The listing builds one solid part. Answer for the finished solid, in the listing's coordinates (mm). Face numbers are marked on the shaded views. A direction names the side the tool comes from. Round coordinates to 2 decimals unless told otherwise and drop trailing zeros. Write each loop counter-clockwise with the first axis right and the second up, starting at its lowest first coordinate (ties: lowest second). Pieces come first, ordered by that corner, then holes. Notation, with made-up numbers: (21.5, 22.25) - (54.5, 22.25) arc R23 cw to (54.5, 43.25) - close; hole circle Ø6 at (82.25, 17.25). An arc over 180 degrees is marked (long way). Return JSON: item names as keys, results as strings. Group by question number.
from build123d import *

# Parameters (mm, degrees)
SKETCH1_W                       = 27.7
SKETCH1_H                       = 41.5
BOSS_EXTRUDE1_DEPTH             = 10
CUT_EXTRUDE2_DEPTH              = 27.877220838
CUT_EXTRUDE2_DEPTH_BACK         = 27.877220838
SKETCH2_R                       = 1.65
BOSS_EXTRUDE2_REACH             = 28.877
SKETCH3_R                       = 1.25
BOSS_EXTRUDE2_DIRECTION_2_REACH = 28.877
CUT_EXTRUDE3_START              = -7
SKETCH4_R                       = 1.25
CUT_EXTRUDE3_DEPTH              = 7
SKETCH6_R                       = 1.25
CUT_EXTRUDE5_DEPTH              = 10
SKETCH5_R                       = 1.25
CUT_EXTRUDE4_DEPTH              = 51.438166105
FILLET1_R                       = 2


with BuildPart() as part:
    # Sketch1 → Boss-Extrude1 (new body)
    with BuildSketch(Plane.XY):
        Rectangle(SKETCH1_W, SKETCH1_H)
    extrude(amount=BOSS_EXTRUDE1_DEPTH)

    # Sketch2 → Cut-Extrude2 (cut, two sides: drawn at the far end of the back side and taken through both)
    with BuildSketch(Plane(origin=(0, 0, 0), x_dir=(0, 0, -1), z_dir=(1, 0, 0)).offset(-CUT_EXTRUDE2_DEPTH_BACK)):
        with Locations((-4, 12.5)):
            Circle(SKETCH2_R)
        with Locations((-4, -12.5)):
            Circle(SKETCH2_R)
    extrude(amount=CUT_EXTRUDE2_DEPTH + CUT_EXTRUDE2_DEPTH_BACK, mode=Mode.SUBTRACT)

    # Boss-Extrude2: up to this face of the body (flat: up to its plane)
    boss_extrude2_end = Plane(part.part.faces().sort_by_distance((-13.85, 0, 5.042991276))[0])
    # Sketch3 → Boss-Extrude2 (add, up to the picked face)
    with BuildSketch(Plane(origin=(0, 0, 0), x_dir=(0, 0, -1), z_dir=(1, 0, 0)), mode=Mode.PRIVATE) as boss_extrude2_sk1:
        Polygon((-15.5, -14.05), (-10, -14.05), (-10, 3.45), (-20.188333796, 3.45), align=None)
    boss_extrude2_tool1 = split(extrude(boss_extrude2_sk1.sketch, amount=-BOSS_EXTRUDE2_REACH, mode=Mode.PRIVATE), bisect_by=boss_extrude2_end, keep=Keep.BOTH, mode=Mode.PRIVATE)
    # Sketch3 → Boss-Extrude2 (add, up to the picked face)
    with BuildSketch(Plane(origin=(0, 0, 0), x_dir=(0, 0, -1), z_dir=(1, 0, 0)), mode=Mode.PRIVATE) as boss_extrude2_sk2:
        with BuildLine():
            Line((-20.188333796, 3.45), (-10, 3.45))
            Line((-10, 3.45), (-10, 20.75))
            Line((-10, 20.75), (-34.754426044, 8.380905804))
            ThreePointArc((-34.754426044, 8.380905804), (-35.758048448, 2.871948872), (-30.188333796, 3.45))
            Line((-30.188333796, 3.45), (-20.188333796, 3.45))
        make_face()
        with Locations(Location((-33.19, 5.25, 0), (0, 0, 90))):
            Circle(SKETCH3_R, mode=Mode.SUBTRACT)
    boss_extrude2_tool2 = split(extrude(boss_extrude2_sk2.sketch, amount=-BOSS_EXTRUDE2_REACH, mode=Mode.PRIVATE), bisect_by=boss_extrude2_end, keep=Keep.BOTH, mode=Mode.PRIVATE)
    # Sketch3 → Boss-Extrude2 (add, up to the picked face)
    with BuildSketch(Plane(origin=(0, 0, 0), x_dir=(0, 0, -1), z_dir=(1, 0, 0)), mode=Mode.PRIVATE) as boss_extrude2_sk3:
        Polygon((-10, -14.05), (-10, -20.75), (-15.5, -14.05), align=None)
    boss_extrude2_tool3 = split(extrude(boss_extrude2_sk3.sketch, amount=-BOSS_EXTRUDE2_REACH, mode=Mode.PRIVATE), bisect_by=boss_extrude2_end, keep=Keep.BOTH, mode=Mode.PRIVATE)
    add(boss_extrude2_tool1.solids().sort_by(Axis((0, -4.428377, 14.038839), (-1, 0, 0)))[0])
    add(boss_extrude2_tool2.solids().sort_by(Axis((0, 9.377547, 20.597774), (-1, 0, 0)))[0])
    add(boss_extrude2_tool3.solids().sort_by(Axis((0, -16.283333, 11.833333), (-1, 0, 0)))[0])

    # Boss-Extrude2 direction 2: up to this face of the body (flat: up to its plane)
    boss_extrude2_direction_2_end = Plane(part.part.faces().sort_by_distance((13.85, 0, 5.042991276))[0])
    # Sketch3 → Boss-Extrude2 direction 2 (add, up to the picked face)
    with BuildSketch(Plane(origin=(0, 0, 0), x_dir=(0, 0, -1), z_dir=(1, 0, 0)), mode=Mode.PRIVATE) as boss_extrude2_direction_2_sk1:
        Polygon((-15.5, -14.05), (-10, -14.05), (-10, 3.45), (-20.188333796, 3.45), align=None)
    boss_extrude2_direction_2_tool1 = split(extrude(boss_extrude2_direction_2_sk1.sketch, amount=BOSS_EXTRUDE2_DIRECTION_2_REACH, mode=Mode.PRIVATE), bisect_by=boss_extrude2_direction_2_end, keep=Keep.BOTH, mode=Mode.PRIVATE)
    # Sketch3 → Boss-Extrude2 direction 2 (add, up to the picked face)
    with BuildSketch(Plane(origin=(0, 0, 0), x_dir=(0, 0, -1), z_dir=(1, 0, 0)), mode=Mode.PRIVATE) as boss_extrude2_direction_2_sk2:
        with BuildLine():
            Line((-20.188333796, 3.45), (-10, 3.45))
            Line((-10, 3.45), (-10, 20.75))
            Line((-10, 20.75), (-34.754426044, 8.380905804))
            ThreePointArc((-34.754426044, 8.380905804), (-35.758048448, 2.871948872), (-30.188333796, 3.45))
            Line((-30.188333796, 3.45), (-20.188333796, 3.45))
        make_face()
        with Locations(Location((-33.19, 5.25, 0), (0, 0, 90))):
            Circle(SKETCH3_R, mode=Mode.SUBTRACT)
    boss_extrude2_direction_2_tool2 = split(extrude(boss_extrude2_direction_2_sk2.sketch, amount=BOSS_EXTRUDE2_DIRECTION_2_REACH, mode=Mode.PRIVATE), bisect_by=boss_extrude2_direction_2_end, keep=Keep.BOTH, mode=Mode.PRIVATE)
    # Sketch3 → Boss-Extrude2 direction 2 (add, up to the picked face)
    with BuildSketch(Plane(origin=(0, 0, 0), x_dir=(0, 0, -1), z_dir=(1, 0, 0)), mode=Mode.PRIVATE) as boss_extrude2_direction_2_sk3:
        Polygon((-10, -14.05), (-10, -20.75), (-15.5, -14.05), align=None)
    boss_extrude2_direction_2_tool3 = split(extrude(boss_extrude2_direction_2_sk3.sketch, amount=BOSS_EXTRUDE2_DIRECTION_2_REACH, mode=Mode.PRIVATE), bisect_by=boss_extrude2_direction_2_end, keep=Keep.BOTH, mode=Mode.PRIVATE)
    add(boss_extrude2_direction_2_tool1.solids().sort_by(Axis((0, -4.428377, 14.038839), (1, 0, 0)))[0])
    add(boss_extrude2_direction_2_tool2.solids().sort_by(Axis((0, 9.377547, 20.597774), (1, 0, 0)))[0])
    add(boss_extrude2_direction_2_tool3.solids().sort_by(Axis((0, -16.283333, 11.833333), (1, 0, 0)))[0])

    # Sketch4 → Cut-Extrude3 (cut)
    # profile 1 of 5: a face of its own
    with BuildSketch(Plane.ZY.offset(13.85).offset(CUT_EXTRUDE3_START)):
        with BuildLine():
            ThreePointArc((34.754426044, 8.380905804), (30.621951552, 7.628051128), (30.188333796, 3.45))
            ThreePointArc((30.188333796, 3.45), (34.123854455, 1.876883361), (36.69, 5.25))
            ThreePointArc((36.69, 5.25), (36.167036375, 7.090449517), (34.754426044, 8.380905804))
        make_face()
        with Locations(Location((33.19, 5.25, 0), (0, 0, 270))):
            Circle(SKETCH4_R, mode=Mode.SUBTRACT)
    # profile 2 of 5: a face of its own
    with BuildSketch(Plane.ZY.offset(13.85).offset(CUT_EXTRUDE3_START)):
        with BuildLine():
            ThreePointArc((29.39, 5.25), (29.505082606, 4.321892356), (29.843359894, 3.45))
            Line((29.843359894, 3.45), (30.188333796, 3.45))
            ThreePointArc((30.188333796, 3.45), (30.621951552, 7.628051128), (34.754426044, 8.380905804))
            Line((34.754426044, 8.380905804), (33.430621051, 9.042374126))
            ThreePointArc((33.430621051, 9.042374126), (30.589457748, 8.020772455), (29.39, 5.25))
        make_face()
    # profile 3 of 5: a face of its own
    with BuildSketch(Plane.ZY.offset(13.85).offset(CUT_EXTRUDE3_START)):
        with BuildLine():
            Line((30.188333796, 3.45), (29.843359894, 3.45))
            ThreePointArc((29.843359894, 3.45), (34.118107644, 1.565082606), (36.99, 5.25))
            ThreePointArc((36.99, 5.25), (35.960772455, 7.850542252), (33.430621051, 9.042374126))
            Line((33.430621051, 9.042374126), (34.754426044, 8.380905804))
            ThreePointArc((34.754426044, 8.380905804), (36.167036375, 7.090449517), (36.69, 5.25))
            ThreePointArc((36.69, 5.25), (34.123854455, 1.876883361), (30.188333796, 3.45))
        make_face()
    # profile 4 of 5: a face of its own
    with BuildSketch(Plane.ZY.offset(13.85).offset(CUT_EXTRUDE3_START)):
        with BuildLine():
            Line((30.188333796, 3.45), (29.843359894, 3.45))
            ThreePointArc((29.843359894, 3.45), (34.118107644, 1.565082606), (36.99, 5.25))
            ThreePointArc((36.99, 5.25), (35.960772455, 7.850542252), (33.430621051, 9.042374126))
            Line((33.430621051, 9.042374126), (34.754426044, 8.380905804))
            ThreePointArc((34.754426044, 8.380905804), (36.167036375, 7.090449517), (36.69, 5.25))
            ThreePointArc((36.69, 5.25), (34.123854455, 1.876883361), (30.188333796, 3.45))
        make_face()
    # profile 5 of 5: a face of its own
    with BuildSketch(Plane.ZY.offset(13.85).offset(CUT_EXTRUDE3_START)):
        with BuildLine():
            Line((29.39, 5.25), (29.39, 3.45))
            Line((29.39, 3.45), (29.843359894, 3.45))
            ThreePointArc((29.843359894, 3.45), (29.505082606, 4.321892356), (29.39, 5.25))
        make_face()
    extrude(amount=CUT_EXTRUDE3_DEPTH, mode=Mode.SUBTRACT)

    # Sketch6 → Cut-Extrude5 (cut)
    # profile 1 of 3: a face of its own
    with BuildSketch(Plane(origin=(13.85, 0, 0), x_dir=(0, 0, -1), z_dir=(1, 0, 0))):
        with BuildLine():
            ThreePointArc((-33.430621051, 9.042374126), (-36.388515387, 3.19829356), (-29.843359894, 3.45))
            Line((-29.843359894, 3.45), (-30.188333796, 3.45))
            ThreePointArc((-30.188333796, 3.45), (-35.758048448, 2.871948872), (-34.754426044, 8.380905804))
            Line((-34.754426044, 8.380905804), (-33.430621051, 9.042374126))
        make_face()
    # profile 2 of 3: a face of its own
    with BuildSketch(Plane(origin=(13.85, 0, 0), x_dir=(0, 0, -1), z_dir=(1, 0, 0))):
        with BuildLine():
            Line((-30.188333796, 3.45), (-29.843359894, 3.45))
            ThreePointArc((-29.843359894, 3.45), (-29.505082606, 4.321892356), (-29.39, 5.25))
            ThreePointArc((-29.39, 5.25), (-30.589457748, 8.020772455), (-33.430621051, 9.042374126))
            Line((-33.430621051, 9.042374126), (-34.754426044, 8.380905804))
            ThreePointArc((-34.754426044, 8.380905804), (-35.758048448, 2.871948872), (-30.188333796, 3.45))
        make_face()
        with Locations(Location((-33.19, 5.25, 0), (0, 0, 90))):
            Circle(SKETCH6_R, mode=Mode.SUBTRACT)
    # profile 3 of 3: a face of its own
    with BuildSketch(Plane(origin=(13.85, 0, 0), x_dir=(0, 0, -1), z_dir=(1, 0, 0))):
        with BuildLine():
            Line((-29.843359894, 3.45), (-29.39, 3.45))
            Line((-29.39, 3.45), (-29.39, 5.25))
            ThreePointArc((-29.39, 5.25), (-29.505082606, 4.321892356), (-29.843359894, 3.45))
        make_face()
    extrude(amount=-CUT_EXTRUDE5_DEPTH, mode=Mode.SUBTRACT)

    # Sketch5 → Cut-Extrude4 (cut, through all)
    with BuildSketch(Plane.ZY.offset(13.85)):
        with Locations(Location((14.5, 12.353095448, 0), (0, 0, 270))):
            Circle(SKETCH5_R)
        with Locations(Location((22.999243301, 8.106261334, 0), (0, 0, 270))):
            Circle(SKETCH5_R)
    extrude(amount=-CUT_EXTRUDE4_DEPTH, mode=Mode.SUBTRACT)

    # Fillet1
    fillet1_edges = [part.edges().sort_by_distance(p)[0] for p in [
        (0, 20.75, 10),
        (0, 3.45, 20.188333796),
        (0, -14.05, 15.5),
        (0, 20.75, 0),
        (0, -20.75, 0),
        (0, -20.75, 10),
    ]]
    fillet(fillet1_edges, radius=FILLET1_R)


solid = part.part
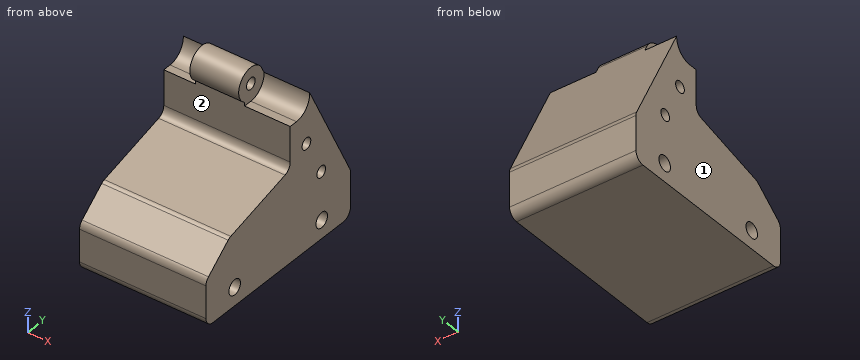
(1) Flat-ended cylindrical pins translate along their axes: pin 1 (6 mm diameter, centred on y = 4.5, z = 32.5, fed in from -X); pin 2 (4 mm diameter, centred on x = -6, z = 25.5, fed in from -Y); pin 3 (10 mm diameter, centred on x = 0.5, z = 15.5, fed in from +Y). Find the tip coordinate at first contact, or state that the pin passes through.
(2) Find section B-B (y = -12.5). Write down the section's boundary in (x, z).
(3) Find section A-A (z = 4). Write down the section's boundary in (x, y), plus the area to 3 significant figures.
(4) Find section C-C (y = 12.5). Write down the section's boundary in (x, z), plus the area to 3 significant figures.
(5) Find section D-D (z = 14.5). Write down the section's boundary in (x, y).
(6) Consider line 1 (Z direction, x = 12, y = 13); line 2 (Z direction, x = -2.75, y = 5.25); line 3 (Z direction, x = -10.25, y = 2). Determine where each line is inside the solid, lowest interval first.
(7) For the marked faces 1 and 2, determine the directions among +Z, -Z, +X, -X, +Y, -Y from which every point of the face is accessible in a straight line to the end or side of a thin tool.
Check sheet entries:
{
 "1": {"pin 1": "stops at x = -6.85", "pin 2": "stops at y = 3.45", "pin 3": "stops at y = 20.5"},
 "2": {"outline": "(-13.85, 0) - (13.85, 0) - (13.85, 2.35) - (-13.85, 2.35) - close; (-13.85, 5.65) - (13.85, 5.65) - (13.85, 15.92) - (-13.85, 15.92) - close"},
 "3": {"outline": "(-13.85, -20.75) - (13.85, -20.75) - (13.85, -14.15) - (-13.85, -14.15) - close; (-13.85, -10.85) - (13.85, -10.85) - (13.85, 10.85) - (-13.85, 10.85) - close; (-13.85, 14.15) - (13.85, 14.15) - (13.85, 20.75) - (-13.85, 20.75) - close", "area": "967 mm^2"},
 "4": {"outline": "(-13.85, 0) - (13.85, 0) - (13.85, 2.35) - (-13.85, 2.35) - close; (-13.85, 5.65) - (13.85, 5.65) - (13.85, 13.26) - (-13.85, 13.26) - close; (-13.85, 15.74) - (13.85, 15.74) - (13.85, 26.51) - (-13.85, 26.51) - close", "area": "574 mm^2"},
 "5": {"outline": "(-13.85, -15.27) - (13.85, -15.27) - (13.85, 11.1) - (-13.85, 11.1) - close; (-13.85, 13.6) - (13.85, 13.6) - (13.85, 18.5) - (-13.85, 18.5) - close"},
 "6": {"line 1": "z = 0 to 2.43, 5.57 to 13.43, 15.57 to 25.51", "line 2": "z = 0 to 31.94, 34.44 to 36.69", "line 3": "z = 0 to 19.8"},
 "7": {"face 1": "+Z, -Z, -X, +Y, -Y", "face 2": "+X, -X, -Y"}
}
